For this review, take the finished solid that the model builds, in its own axes (mm). A direction names the side the tool comes from. Give positions to 0.01 mm unless a question says otherwise; leave off trailing zeros. Loops run counter-clockwise (first coordinate to the right, second up) from the corner with the lowest first, then second, coordinate; pieces in that order, holes last. Notation, with made-up numbers: M -18.75,-10.75 L -4.75,-10.75 A13 ccw -4.75,1.25 Z; hole C 28.25,29.5 d8. An arc over 180 degrees is marked long. Use CSV: the item, a comma, the result in double quotes. Start each with the question number.
1. Take a section at B-B, the plane x = 18.5. Write out the cut boundary in (y, z) (3 decimals), and give its area (3 significant figures).
2. Insertion check: P1, Ø3, axis at x = 3, y = 1.5, coming from the +Z side; P2, Ø0.6, axis at x = 16, y = 4.5, coming from the +Z side; P3, Ø1.6, axis at x = 18, y = 4, coming from the -Z side. Each pin has a flat end and moves straight along its axis. Give the tip position at first contact, or say it passes through.
3. Tool access review of faces 1 (the face through (18, 4, -3.175)), 2 (the face through (18, 3.048, 5)), 3 (the face through (18, 3.048, -5)), 4 (the face through (-3, 0, -5.563)): name each direction out of +Z, -Z, +X, -X, +Y, -Y from which nothing blocks a thin tool from reaching the whole face with its end or side.
4. To check wall thickness, follow line 1 (Z direction, x = 6.5, y = 1.5); line 2 (X direction, y = -2, z = -3.25); line 3 (Y direction, x = -12, z = 2). State the ranges of each line that lie inside material, in increasing order. Write a range as [from, to].
5. Take a section at A-A, the plane y = 3.75. Write out the cut boundary in (x, z) (3 decimals).
6. The part is to be moulded in two halves that separate along Z. For faces 5 (the face through (23, -1.27, 0)), 6 (the face through (23, 0, 1.714)), 7 (the face through (18, 3.048, 0)), say which applies: pulls with the +Z half, pulls with the -Z half, needs draft (parallel to the pull), parting line crosses it, or undercut.
7. Take a section at D-D, the plane z = 1.25. Write out the cut boundary in (x, y) (3 decimals).
from build123d import *

# Parameters (mm, degrees)
SKETCH1_W           = 41.91
SKETCH1_H           = 12.7
BOSS_EXTRUDE1_DEPTH = 3.048
SKETCH2_W           = 0.762
SKETCH2_H           = 2.032
BOSS_EXTRUDE2_DEPTH = 6.604
SKETCH2_3_W         = 3.429
SKETCH2_3_H         = 1.27
BOSS_EXTRUDE3_DEPTH = 3.175
CUT_EXTRUDE1_START  = -6.604
SKETCH4_W           = 14.239901434
SKETCH4_H           = 7.9172944
SKETCH4_W_2         = 11.1252
SKETCH4_H_2         = 5.4356
CUT_EXTRUDE1_DEPTH  = 36.306
FILLET1_R           = 0.762
CUT_EXTRUDE2_DEPTH  = 0.127
SKETCH6_W           = 3.429
SKETCH6_H           = 2.54
BOSS_EXTRUDE4_DEPTH = 0.127


with BuildPart() as part:
    # Sketch1 → Boss-Extrude1 (new body, symmetric)
    with BuildSketch(Plane(origin=(0, 0, 0), x_dir=(1, 0, 0), z_dir=(0, 1, 0))):
        Rectangle(SKETCH1_W, SKETCH1_H)
    extrude(amount=BOSS_EXTRUDE1_DEPTH, both=True)

    # Sketch2 → Boss-Extrude2 (add)
    with BuildSketch(Plane(origin=(20.955, 0, 0), x_dir=(0, 0, -1), z_dir=(1, 0, 0))):
        with Locations((-3.556, 4.064)):
            Rectangle(SKETCH2_W, SKETCH2_H)
        with Locations((3.556, 4.064)):
            Rectangle(SKETCH2_W, SKETCH2_H)
    extrude(amount=-BOSS_EXTRUDE2_DEPTH)

    # Sketch2<3> → Boss-Extrude3 (add)
    with BuildSketch(Plane(origin=(20.955, 0, 0), x_dir=(0, 0, -1), z_dir=(1, 0, 0))):
        with Locations((0, 0.635)):
            Rectangle(SKETCH2_3_W, SKETCH2_3_H)
        with Locations((0, -0.635)):
            Rectangle(SKETCH2_3_W, SKETCH2_3_H)
    extrude(amount=BOSS_EXTRUDE3_DEPTH)

    # Sketch4 → Cut-Extrude1 (cut, through all)
    with BuildSketch(Plane(origin=(20.955, 0, 0), x_dir=(0, 0, -1), z_dir=(1, 0, 0)).offset(CUT_EXTRUDE1_START)):
        Rectangle(SKETCH4_W, SKETCH4_H)
        Rectangle(SKETCH4_W_2, SKETCH4_H_2, mode=Mode.SUBTRACT)
    extrude(amount=-CUT_EXTRUDE1_DEPTH, mode=Mode.SUBTRACT)

    # Fillet1
    fillet1_edges = [part.edges().sort_by_distance(p)[0] for p in [
        (-20.955, 0, 5.5626),
        (-20.955, -2.7178, 0),
        (-20.955, 0, -5.5626),
        (-20.955, 2.7178, 0),
        (-3.302, -2.7178, 5.5626),
        (-3.302, 2.7178, 5.5626),
        (-3.302, 2.7178, -5.5626),
        (-3.302, -2.7178, -5.5626),
    ]]
    fillet(fillet1_edges, radius=FILLET1_R)

    # Sketch5 → Cut-Extrude2 (cut)
    with BuildSketch(Plane(origin=(20.955, 0, 0), x_dir=(0, 0, -1), z_dir=(1, 0, 0))):
        Polygon((-6.35, -3.048), (6.35, -3.048), (6.35, 3.048), (3.937, 3.048), (3.937, 5.08), (3.175, 5.08), (3.175, 3.048), (-3.175, 3.048), (-3.175, 5.08), (-3.937, 5.08), (-3.937, 3.048), (-6.35, 3.048), align=None)
    extrude(amount=-CUT_EXTRUDE2_DEPTH, mode=Mode.SUBTRACT)

    # Sketch6 → Boss-Extrude4 (add)
    with BuildSketch(Plane.ZY.offset(-20.955)):
        Rectangle(SKETCH6_W, SKETCH6_H)
    extrude(amount=BOSS_EXTRUDE4_DEPTH)


solid = part.part
Result set:
1,outline,"M -3.048,-6.35 L 3.048,-6.35 L 3.048,-3.937 L 5.08,-3.937 L 5.08,-3.175 L 3.048,-3.175 L 3.048,3.175 L 5.08,3.175 L 5.08,3.937 L 3.048,3.937 L 3.048,6.35 L -3.048,6.35 Z"
1,area,"80.5 mm2"
2,P1,"z = 5.56"
2,P2,"z = 3.94"
2,P3,"z = -3.94"
3,face 1,"+X, -X, +Y"
3,face 2,"+Z, +X, -X, +Y"
3,face 3,"-Z, +X, -X, +Y"
3,face 4,"-Z, -X, +Y, -Y"
4,line 1,"[-5.56, 5.56]"
4,line 2,"[-20.95, 20.83]"
4,line 3,"[-2.72, 2.72]"
5,outline,"M 14.351,-3.937 L 20.828,-3.937 L 20.828,-3.175 L 14.351,-3.175 Z; M 14.351,3.175 L 20.828,3.175 L 20.828,3.937 L 14.351,3.937 Z"
6,face 5,"needs draft"
6,face 6,"pulls with the +Z half"
6,face 7,"undercut"
7,outline,"M -20.955,-1.956 A0.762 ccw -20.193,-2.718 L 14.351,-2.718 L 14.351,-3.048 L 20.828,-3.048 L 20.828,-1.27 L 24.13,-1.27 L 24.13,1.27 L 20.828,1.27 L 20.828,3.048 L 14.351,3.048 L 14.351,2.718 L -20.193,2.718 A0.762 ccw -20.955,1.956 Z"
